Design review of the part shown in the three views and the two pictorial views. Dimensions are in mm from the part's minimum x, y and z. A direction names the side the tool comes from. Give positions to 0.01 mm unless a question says otherwise; leave off trailing zeros. Loops run counter-clockwise (first coordinate to the right, second up) from the corner with the lowest first, then second, coordinate; pieces in that order, holes last.
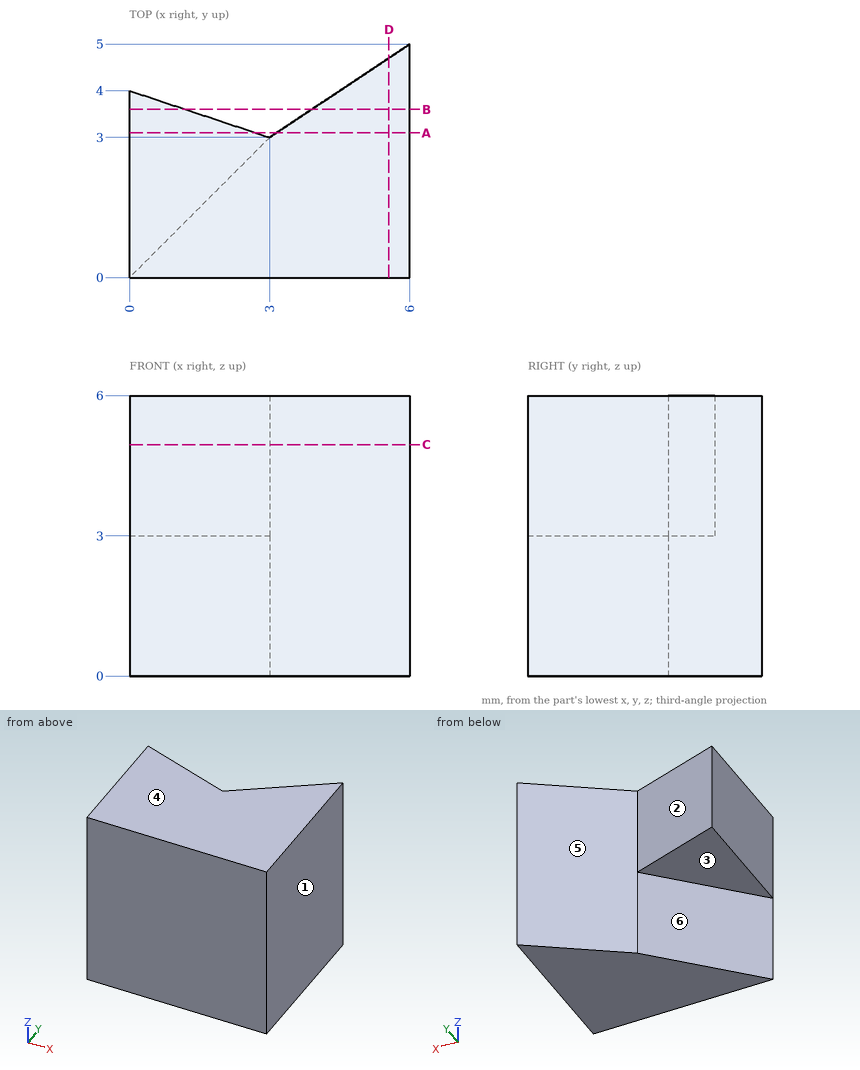
Q1. Take a section at B-B (y = 3.6). Give the boundary of the cut face in (x, z).
Results:
outline: (0, 3) - (1.2, 3) - (1.2, 6) - (0, 6) - close; (3.9, 0) - (6, 0) - (6, 6) - (3.9, 6) - close
Q2. Draft analysis for pull direction X (two halves, no side actions). For the marked faces 1, 2 and 3, state which applies: pulls with the +X half, pulls with the -X half, needs draft (parallel to the pull), parting line crosses it, or undercut.
Results:
face 1: pulls with the +X half
face 2: undercut
face 3: needs draft
Q3. Take a section at D-D (x = 5.55). Give the boundary of the cut face in (y, z), plus the area to 3 significant figures.
Results:
outline: (0, 0) - (4.7, 0) - (4.7, 6) - (0, 6) - close
area: 28.2 mm2
Q4. Take a section at C-C (z = 4.95). Give the boundary of the cut face in (x, y), plus the area to 3 significant figures.
Results:
outline: (0, 0) - (6, 0) - (6, 5) - (3, 3) - (0, 4) - close
area: 22.5 mm2
Q5. Insertion check: pin 1 (1 mm diameter, centred on x = 1.5, z = 5.5, fed in from +Y). The pin has a flat end and moves straight along its axis. Give the tip position at first contact, or say it passes through.
Results:
pin 1: stops at y = 3.67
Q6. Take a section at A-A (y = 3.1). Give the boundary of the cut face in (x, z).
Results:
outline: (0, 3) - (2.7, 3) - (2.7, 6) - (0, 6) - close; (3.15, 0) - (6, 0) - (6, 6) - (3.15, 6) - close
Q7. Tool access review of the marked faces 4, 5 and 6: name each direction out of +Z, -Z, +X, -X, +Y, -Y from which nothing blocks a thin tool from reaching the whole face with its end or side.
Results:
face 4: +Z, +X, -X, +Y, -Y
face 5: +Z, -Z, +Y
face 6: -Z, -X, +Y
Q8. Wall thickness on line 1 (Z direction, x = 0.75, y = 0.95); line 2 (Y direction, x = 0.7, z = 0.45); line 3 (X direction, y = 4.65, z = 3.55) (3 decimals): over which ranges is each line inside the solid? List them lowest first.
Results:
line 1: z = 3 to 6
line 2: y = 0 to 0.7
line 3: x = 5.475 to 6
